For this review, take the finished solid that the model builds, in its own axes (mm). Face numbers are marked on the shaded views. Give positions to 0.01 mm unless a question says otherwise; leave off trailing zeros. Loops run counter-clockwise (first coordinate to the right, second up) from the corner with the lowest first, then second, coordinate; pieces in that order, holes last. Notation, with made-up numbers: (-13.75, 53.25) - (-6.75, 53.25) arc R12 cw to (-6.75, 65.25) - close; hole circle Ø2 at (-26, 35). An arc over 180 degrees is marked (long way). Put each result on its own line as item: value.
from build123d import *

# Parameters (mm, degrees)
SKETCH1_R                = 17.5
BOSS_EXTRUDE1_DEPTH      = 100
SKETCH2_R                = 12.5
CUT_EXTRUDE1_DEPTH       = 90
SKETCH3_W                = 20
SKETCH3_H                = 15
SKETCH3_R                = 4.15
BOSS_EXTRUDE2_DEPTH      = 5
BOSS_EXTRUDE2_DEPTH_BACK = 5
FILLET1_R                = 3


with BuildPart() as part:
    # Sketch1 → Boss-Extrude1 (new body)
    with BuildSketch(Plane.XY):
        Circle(SKETCH1_R)
    extrude(amount=BOSS_EXTRUDE1_DEPTH)

    # Sketch2 → Cut-Extrude1 (cut)
    with BuildSketch(Plane.XY.offset(100)):
        Circle(SKETCH2_R)
    extrude(amount=-CUT_EXTRUDE1_DEPTH, mode=Mode.SUBTRACT)

    # Sketch3 → Boss-Extrude2 (add, two sides)
    with BuildSketch(Plane(origin=(0, 0, 0), x_dir=(0, 0, -1), z_dir=(1, 0, 0))) as boss_extrude2_sk:
        with Locations((10, 0)):
            Rectangle(SKETCH3_W, SKETCH3_H)
        with Locations((12.5, 0)):
            Circle(SKETCH3_R, mode=Mode.SUBTRACT)
    extrude(amount=BOSS_EXTRUDE2_DEPTH)
    extrude(boss_extrude2_sk.sketch, amount=-BOSS_EXTRUDE2_DEPTH_BACK)

    # Fillet1
    fillet1_edges = [part.edges().sort_by_distance(p)[0] for p in [
        (0, 7.5, 0),
        (0, 7.5, -20),
        (0, -7.5, -20),
        (0, -7.5, 0),
        (-5, 0, 0),
        (5, 0, 0),
        (-17.5, 0, 0),
    ]]
    fillet(fillet1_edges, radius=FILLET1_R)


solid = part.part
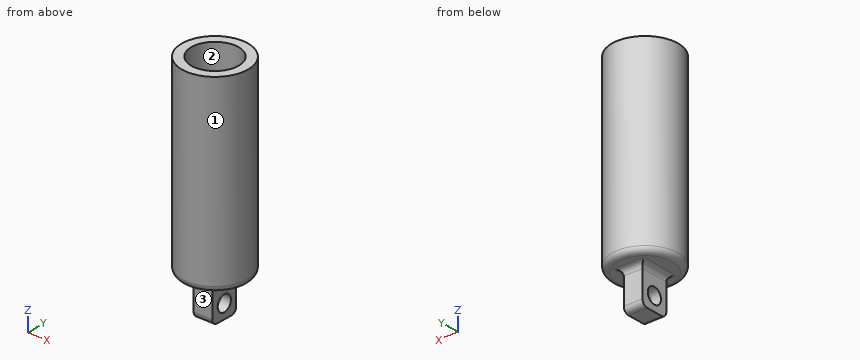
1) Wall thickness on line 1 (Y direction, x = -2.4, z = -12.5); line 2 (Y direction, x = 0, z = 83.5); line 3 (Z direction, x = -13, y = 2): over which ranges is each line inside the solid? List them lowest first.
Geometry check:
line 1: y = -7.5 to -4.15, 4.15 to 7.5
line 2: y = -17.5 to -12.5, 12.5 to 17.5
line 3: z = 0 to 100
2) Take a section at C-C on z = 64. State the section outline as (x, y) points.
Geometry check:
outline: circle Ø35 at (0, 0); hole circle Ø25 at (0, 0)
3) Insertion check: pin 1 Ø2 at (x, y) = (-7.5, -9) entering from -Z; pin 2 Ø10 at (x, z) = (13.5, 59.5) entering from -Y; pin 3 Ø9.5 at (y, z) = (0, -12.5) entering from -X; pin 4 Ø6.5 at (y, z) = (0, -12.5) entering from -X. Each pin has a flat end and moves straight along its axis. Give the tip position at first contact, or say it passes through.
Geometry check:
pin 1: stops at z = -0.4
pin 2: stops at y = -15.3
pin 3: stops at x = -5
pin 4: passes through
4) Take a section at A-A on y = 0. State the section outline as (x, z) points.
Geometry check:
outline: (-17.5, 3) arc R3 ccw to (-14.5, 0) - (-8, 0) arc R3 cw to (-5, -3) - (-5, -8.35) - (5, -8.35) - (5, -3) arc R3 cw to (8, 0) - (14.5, 0) arc R3 ccw to (17.5, 3) - (17.5, 100) - (12.5, 100) - (12.5, 10) - (-12.5, 10) - (-12.5, 100) - (-17.5, 100) - close; (-5, -20) - (5, -20) - (5, -16.65) - (-5, -16.65) - close
5) Draft analysis for pull direction X (two halves, no side actions). For the marked faces 1, 2 and 3, state which applies: pulls with the +X half, pulls with the -X half, needs draft (parallel to the pull), parting line crosses it, or undercut.
Geometry check:
face 1: parting line crosses it
face 2: undercut
face 3: needs draft
6) Take a section at B-B on z = -12.5. State the section outline as (x, y) points, and give its area (3 significant figures).
Geometry check:
outline: (-5, -7.5) - (5, -7.5) - (5, -4.15) - (-5, -4.15) - close; (-5, 4.15) - (5, 4.15) - (5, 7.5) - (-5, 7.5) - close
area: 67.0 mm²
